Source: three-view drawing plus pictorial views. Frame: mm from the lowest corner of the part. Round coordinates to 2 decimals unless told otherwise and drop trailing zeros. Order: outer loops, then holes, each group sorted by start corner. A loop starts at its lowest first (then second) coordinate and runs counter-clockwise, first axis right, second up. Notation, with made-up numbers: M 13.5,-24.5 L 70.5,-24.5 A19 cw 70.5,0.5 Z; hole C 23,38.25 d1. An arc over 180 degrees is marked long. Return JSON: item names as keys, results as strings. Group by question number.
Q1. Cut plane A-A on x = 32. Output: boundary loops of the cut face in (y, z).
Q2. Cut plane C-C on x = 24. Output: boundary loops of the cut face in (y, z), and give its area (3 significant figures).
Q3. Cut plane B-B on y = 23.5. Output: boundary loops of the cut face in (x, z).
Q4. Ray query, probe 1 along Y at (x, z) = (32, 0.7); probe 2 along X at (y, z) = (45.5, 0.3) (1 decimal); probe 3 along Y at (x, z) = (7.5, 0.5) (1 decimal). Return the intervals inside material, ascending.
Q5. Cut plane D-D on z = 0.35. Output: boundary loops of the cut face in (x, y), and give its area (3 significant figures).
Q6. Contact query for a flat-ended pin moving along its axis: pin 1 (2 mm diameter, centred on x = 50, y = 34.5, fed in from -Z). Output: stop coordinate, or through.
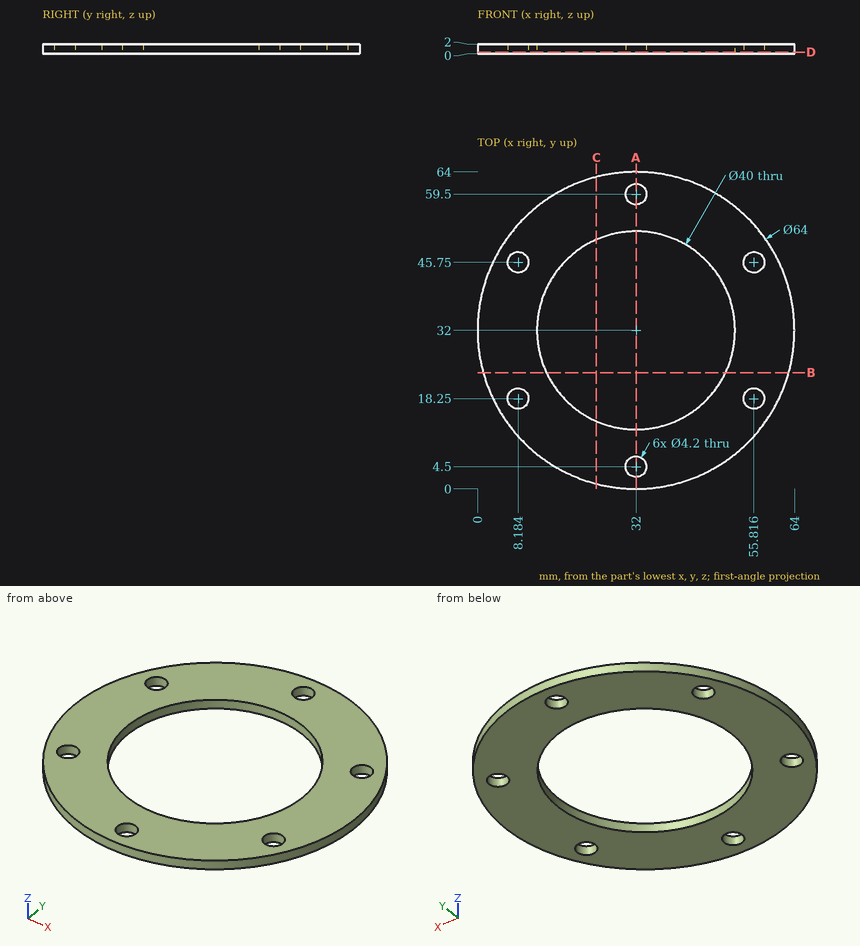
Result sheet:
{
 "1": {"outline": "M 0,0 L 2.4,0 L 2.4,2 L 0,2 Z; M 6.6,0 L 12,0 L 12,2 L 6.6,2 Z; M 52,0 L 57.4,0 L 57.4,2 L 52,2 Z; M 61.6,0 L 64,0 L 64,2 L 61.6,2 Z"},
 "2": {"outline": "M 1.02,0 L 13.67,0 L 13.67,2 L 1.02,2 Z; M 50.33,0 L 62.98,0 L 62.98,2 L 50.33,2 Z", "area": "50.6 mm²"},
 "3": {"outline": "M 1.15,0 L 13.9,0 L 13.9,2 L 1.15,2 Z; M 50.1,0 L 62.85,0 L 62.85,2 L 50.1,2 Z"},
 "4": {"probe 1": "y = 0 to 2.4, 6.6 to 12, 52 to 57.4, 61.6 to 64", "probe 2": "x = 3 to 6.1, 10.3 to 17.2, 46.8 to 53.7, 57.9 to 61", "probe 3": "y = 11.4 to 16.3, 20.2 to 43.8, 47.7 to 52.6"},
 "5": {"outline": "C 32,32 d64; hole C 8.18,18.25 d4.2; hole C 8.18,45.75 d4.2; hole C 32,32 d40; hole C 32,4.5 d4.2; hole C 32,59.5 d4.2; hole C 55.82,18.25 d4.2; hole C 55.82,45.75 d4.2", "area": "1,880 mm²"},
 "6": {"pin 1": "passes through"}
}
